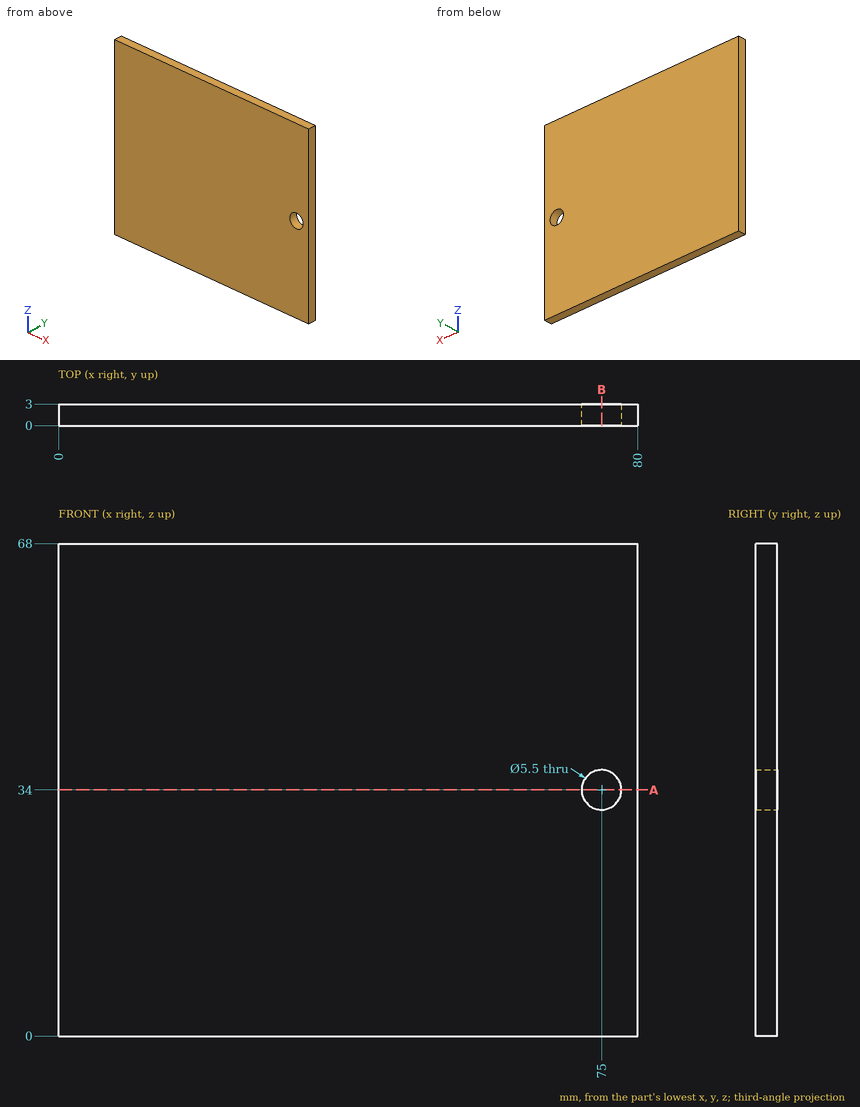
Here's the drawing with two shaded views (mm, measured from the low corner). I have some questions. Round coordinates to 2 decimals unless told otherwise and drop trailing zeros. Loops run counter-clockwise (first coordinate to the right, second up) from the corner with the lowest first, then second, coordinate; pieces in that order, holes last. Notation, with made-up numbers: M -37.75,-13.5 L 11.25,-13.5 A13 cw 11.25,-1.5 Z; hole C 6.5,72.5 d4. An arc over 180 degrees is marked long. Answer as a JSON object with one key per item and string values. Group by question number.
Q1. Will this pin go through, and if not, where does the flat tip stop? pin 1 (1 mm diameter, centred on x = 66.5, z = 38, fed in from -Y).
Q2. Imagine slicing it at B-B, the plane x = 75. Please give me the cut outline in (y, z), then the cut area to 4 significant figures.
Q3. Please list where this line runs through material, in increasing order: L1, parallel to Z at x = 75, y = 2.1.
Q4. Imagine slicing it at A-A, the plane z = 34. Please give me the cut outline in (x, y).
Findings:
{
 "1": {"pin 1": "stops at y = 0"},
 "2": {"outline": "M 0,0 L 3,0 L 3,31.25 L 0,31.25 Z; M 0,36.75 L 3,36.75 L 3,68 L 0,68 Z", "area": "187.5 mm2"},
 "3": {"L1": "z = 0 to 31.25, 36.75 to 68"},
 "4": {"outline": "M 0,0 L 72.25,0 L 72.25,3 L 0,3 Z; M 77.75,0 L 80,0 L 80,3 L 77.75,3 Z"}
}
